Check sheet for the modelled part. Datum: model origin and axes. Units: mm. Face numbers are marked on the shaded views. Round coordinates to 2 decimals unless told otherwise and drop trailing zeros. Loops run counter-clockwise (first coordinate to the right, second up) from the corner with the lowest first, then second, coordinate; pieces in that order, holes last. Notation, with made-up numbers: M 85.25,56 L 128.25,56 A26 ccw 128.25,90 Z; hole C -35,-18 d10. An arc over 180 degrees is marked long. Write item = value, one per line. Start each with the question number.
(1) Cross-section at D-D on x = -6. Record the boundary of the cut face in (y, z), plus the area to 3 significant figures.
(2) Cross-section at C-C on z = 26. Record the boundary of the cut face in (x, y).
(3) Cross-section at A-A on z = 10.5. Record the boundary of the cut face in (x, y).
(4) Go/stop test with flat-tipped pins: P1, Ø8, axis at y = 16, z = 18.5, coming from the +X side (3 decimals); P2, Ø4, axis at x = -10.5, y = 13, coming from the -Z side; P3, Ø3, axis at x = -11.5, y = 6, coming from the -Z side. Record where each tip stops, or that it passes through.
(5) Mould release check, pull along Y, two halves, no side actions. Record for the marked faces 1 and 2: pulls with the +Y half, pulls with the -Y half, needs draft (parallel to the pull), parting line crosses it, or undercut.
(6) Cross-section at B-B on x = -9.5. Record the boundary of the cut face in (y, z), plus the area to 3 significant figures.
(7) Scan lines: L1, parallel to Y at x = -12.75, z = 21; L2, parallel to Y at x = -8, z = 25; L3, parallel to Z at x = -9.5, y = 4.5. Record each from-to range of solid material in increasing order. Write a range as from..to.
from build123d import *
from build123d.topology import SkipClean

# Parameters (mm, degrees)
BOSS_EXTRUDE1_DEPTH = 3
FILLET1_R           = 1
SKETCH2_R           = 3
BOSS_EXTRUDE2_DEPTH = 12


with BuildPart() as part:
    # Sketch1 → Boss-Extrude1 (new body)
    with BuildSketch(Plane(origin=(0, 0, 0), x_dir=(1, 0, 0), z_dir=(0, 1, 0))):
        with BuildLine():
            Line((-13.284983977, -5.078381136), (-1.284983977, -5.078381136))
            ThreePointArc((-1.284983977, -5.078381136), (0.129229585, -5.664167574), (0.715016023, -7.078381136))
            Line((0.715016023, -7.078381136), (0.715016023, -36.078381136))
            ThreePointArc((0.715016023, -36.078381136), (0.129229585, -37.492594699), (-1.284983977, -38.078381136))
            Line((-1.284983977, -38.078381136), (-13.284983977, -38.078381136))
            ThreePointArc((-13.284983977, -38.078381136), (-14.69919754, -37.492594699), (-15.284983977, -36.078381136))
            Line((-15.284983977, -36.078381136), (-15.284983977, -7.078381136))
            ThreePointArc((-15.284983977, -7.078381136), (-14.69919754, -5.664167574), (-13.284983977, -5.078381136))
        make_face()
    extrude(amount=BOSS_EXTRUDE1_DEPTH)

    # Fillet1
    fillet1_edges = [part.edges().sort_by_distance(p)[0] for p in [
        (-14.69919754, 3, 5.664167574),
        (-15.284983977, 3, 21.578381136),
        (-14.69919754, 3, 37.492594699),
        (-7.284983977, 3, 38.078381136),
        (0.129229585, 3, 37.492594699),
        (0.715016023, 3, 21.578381136),
        (0.129229585, 3, 5.664167574),
        (-7.284983977, 3, 5.078381136),
    ]]
    fillet(fillet1_edges, radius=FILLET1_R)

    # Sketch2 → Boss-Extrude2 (add)
    with BuildSketch(Plane(origin=(0, 3, 0), x_dir=(1, 0, 0), z_dir=(0, 1, 0))):
        with Locations(Location((-7.284983977, -21.578381136, 0), (0, 0, 90))):
            Circle(SKETCH2_R)
    extrude(amount=BOSS_EXTRUDE2_DEPTH)

    # Sketch3 → Revolve9 (revolve)
    with SkipClean():  # the faces are left unmerged after this step: merging them gives an invalid solid
        with BuildSketch(Plane(origin=(0, 15, 0), x_dir=(1, 0, 0), z_dir=(0, 1, 0))):
            with BuildLine():
                ThreePointArc((-2.284983977, -21.578381136), (-3.749450071, -18.04284723), (-7.284983977, -16.578381136))
                Line((-7.284983977, -16.578381136), (-7.284983977, -18.578381136))
                ThreePointArc((-7.284983977, -18.578381136), (-5.163663634, -19.457060793), (-4.284983977, -21.578381136))
                ThreePointArc((-4.284983977, -21.578381136), (-5.163663634, -23.69970148), (-7.284983977, -24.578381136))
                Line((-7.284983977, -24.578381136), (-7.284983977, -26.578381136))
                ThreePointArc((-7.284983977, -26.578381136), (-3.749450071, -25.113915042), (-2.284983977, -21.578381136))
            make_face()
            with BuildLine():
                Line((-7.284983977, -18.578381136), (-7.284983977, -16.578381136))
                ThreePointArc((-7.284983977, -16.578381136), (-12.284983977, -21.578381136), (-7.284983977, -26.578381136))
                Line((-7.284983977, -26.578381136), (-7.284983977, -24.578381136))
                ThreePointArc((-7.284983977, -24.578381136), (-10.284983977, -21.578381136), (-7.284983977, -18.578381136))
            make_face()
        revolve(axis=Axis((-7.284983977, 15, 12.733179874), (0, 0, 1)))


solid = part.part
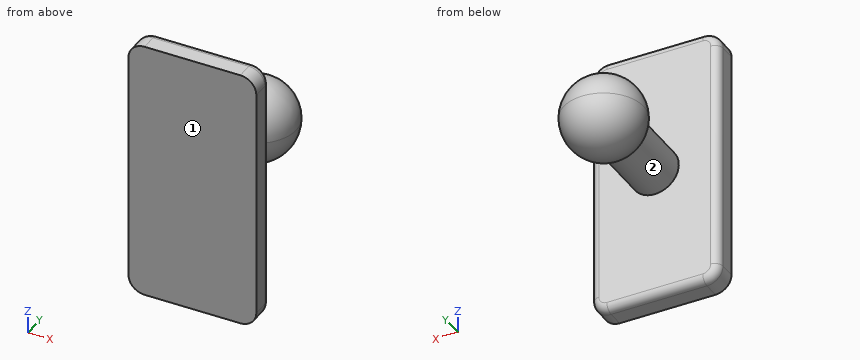
Result:
q1.outline = M 0,5.08 L 2,5.08 A1 ccw 3,6.08 L 3,18.87 L 11,18.87 A4.83 ccw long 11,24.29 L 3,24.29 L 3,37.08 A1 ccw 2,38.08 L 0,38.08 Z; hole M 15,18.87 A2.71 ccw 15,24.29 Z
q1.area = 201 mm^2
q2.outline = M -15.28,0 L 0.72,0 L 0.72,2 A1 ccw -0.28,3 L -14.28,3 A1 ccw -15.28,2 Z; C -7.28,15 d4.67
q3.outline = M -15.28,0 L 0.72,0 L 0.72,2 A1 ccw -0.28,3 L -14.28,3 A1 ccw -15.28,2 Z
q4.P1 = -2.285
q4.P2 = 16.91
q4.P3 = 20.3
q5.face_1 = pulls with the -Y half
q5.face_2 = undercut
q6.outline = M 0,5.08 L 2,5.08 A1 ccw 3,6.08 L 3,19.56 L 11,19.56 A4.48 ccw long 11,23.6 L 3,23.6 L 3,37.08 A1 ccw 2,38.08 L 0,38.08 Z; hole M 15,19.56 A2.02 ccw 15,23.6 Z
q6.area = 186 mm^2
q7.L1 = 0..3
q7.L2 = 0..3, 11.42..18.58
q7.L3 = 19.56..23.6
